from build123d import *

# Parameters (mm, degrees)
SKETCH1_W           = 482.6
SKETCH1_H           = 304.8
BOSS_EXTRUDE1_DEPTH = 6.35
SKETCH2_R           = 2.7813
CUT_EXTRUDE1_DEPTH  = 286.467638271
SKETCH3_R           = 3.175
CUT_EXTRUDE2_DEPTH  = 286.467638271
SKETCH4_R           = 12.7
CUT_EXTRUDE3_DEPTH  = 286.467638271


with BuildPart() as part:
    # Sketch1 → Boss-Extrude1 (new body)
    with BuildSketch(Plane.XY):
        Rectangle(SKETCH1_W, SKETCH1_H)
    extrude(amount=BOSS_EXTRUDE1_DEPTH)

    # Sketch2 → Cut-Extrude1 (cut, through all)
    with BuildSketch(Plane.XY.offset(6.35)):
        with Locations((-232.5624, 146.05)):
            Circle(SKETCH2_R)
        with Locations((-232.5624, -107.95)):
            Circle(SKETCH2_R)
    cut_extrude1 = extrude(amount=-CUT_EXTRUDE1_DEPTH, mode=Mode.SUBTRACT)

    # Mirror1: Cut-Extrude1 across plane
    add(cut_extrude1.mirror(Plane(origin=(0, 0, 0), x_dir=(0, 0, 1), z_dir=(1, 0, 0))), mode=Mode.SUBTRACT)

    # Sketch3 → Cut-Extrude2 (cut, through all)
    with BuildSketch(Plane.XY.offset(6.35)):
        with Locations((-234.95, -139.7)):
            Circle(SKETCH3_R)
        with Locations((-209.55, -139.7)):
            Circle(SKETCH3_R)
    cut_extrude2 = extrude(amount=-CUT_EXTRUDE2_DEPTH, mode=Mode.SUBTRACT)

    # Mirror2: Cut-Extrude2 across plane
    add(cut_extrude2.mirror(Plane(origin=(0, 0, 0), x_dir=(0, 0, 1), z_dir=(1, 0, 0))), mode=Mode.SUBTRACT)

    # Sketch4 → Cut-Extrude3 (cut, through all)
    with BuildSketch(Plane.XY.offset(6.35)):
        with Locations((196.469, -12.7)):
            Circle(SKETCH4_R)
    extrude(amount=-CUT_EXTRUDE3_DEPTH, mode=Mode.SUBTRACT)


solid = part.part
Design review of the part built by this model. Coordinates are the model's own, in mm. Coordinates: 2 decimals unless noted, no trailing zeros. Order: outer loops, then holes, each group sorted by start corner. A loop starts at its lowest first (then second) coordinate and runs counter-clockwise, first axis right, second up. Notation, with made-up numbers: (9.25, -6) -> (63.25, -6) arc R15 cw to (63.25, 20) -> close; hole circle Ø3 at (86.5, -33). An arc over 180 degrees is marked (long way). Use one line per item in the form item = value. Start each with the question number.
(1) Add section A-A on y = -12.7. State the section outline as (x, z) points.
(2) The part is to be moulded in two halves that separate along Y. For faces 1 (the cylindrical face through (208.201, -17.564, 3.219)), 2 (the flat face through (-3, 2, 0)), say which applies: +Y half, -Y half, draft (parallel to the pull), parting line (faces both ways), or undercut.
(3) For probe 1 along X at (y, z) = (146.05, 4); probe 2 along X at (y, z) = (-139.7, 2.75) (3 decimals); probe 3 along Y at (x, z) = (209.55, 4.25) (3 decimals), list the stretches that pass through material, from the lowest coordinate up.
Answer block:
q1.outline = (-241.3, 0) -> (183.77, 0) -> (183.77, 6.35) -> (-241.3, 6.35) -> close; (209.17, 0) -> (241.3, 0) -> (241.3, 6.35) -> (209.17, 6.35) -> close
q2.face_1 = undercut
q2.face_2 = draft
q3.probe_1 = -241.3 to -235.34, -229.78 to 229.78, 235.34 to 241.3
q3.probe_2 = -241.3 to -238.125, -231.775 to -212.725, -206.375 to 206.375, 212.725 to 231.775, 238.125 to 241.3
q3.probe_3 = -152.4 to -142.875, -136.525 to 152.4
